Answer from the drawing. Dimensions are ordinates in mm from the lowest x, y and z of the part. A direction names the side the tool comes from. Coordinates: 2 decimals unless noted, no trailing zeros. Order: outer loops, then holes, each group sorted by start corner. A loop starts at its lowest first (then second) coordinate and runs counter-clockwise, first axis right, second up. Notation, with made-up numbers: (58.5, 7) - (73.5, 7) arc R26 cw to (73.5, 31) - close; hole circle Ø3 at (-13, -39.75). An arc over 180 degrees is marked (long way). Answer as a JSON object with one key per item and string values. Group by question number.
1) Find the intervals of material crossed by line 1 along X through (y, z) = (41, 22.5); line 2 along Y through (x, z) = (53.5, 13.75); line 3 along Y through (x, z) = (77, 10.5), in increasing order.
2) Section C-C (y = 30) is taken. Give the vertices of the cut face in (x, z), plus the area to 3 significant figures.
3) Section D-D (x = 12) is taken. Give the vertices of the cut face in (y, z), plus the area to 3 significant figures.
4) Each of these flat-tipped pins is pushed along its axis until it touches: P1, Ø6, axis at y = 51, z = 10.5, coming from the +X side; P2, Ø1.5, axis at x = 78, z = 7, coming from the +Y side; P3, Ø10, axis at x = 20.5, z = 18.5, coming from the +Y side. Where does it stop, or does it pass through?
5) A tool of negligible diameter and unlimited length cuts with its end or side. For the marked faces 1, 2 and 3, from which of +Z, -Z, +X, -X, +Y, -Y can it reach the whole face along a straight path? Write none if from no direction.
6) Section B-B (x = 44) is taken. Give the vertices of the cut face in (y, z).
7) Section A-A (z = 15) is taken. Give the vertices of the cut face in (x, y), plus the area to 3 significant figures.
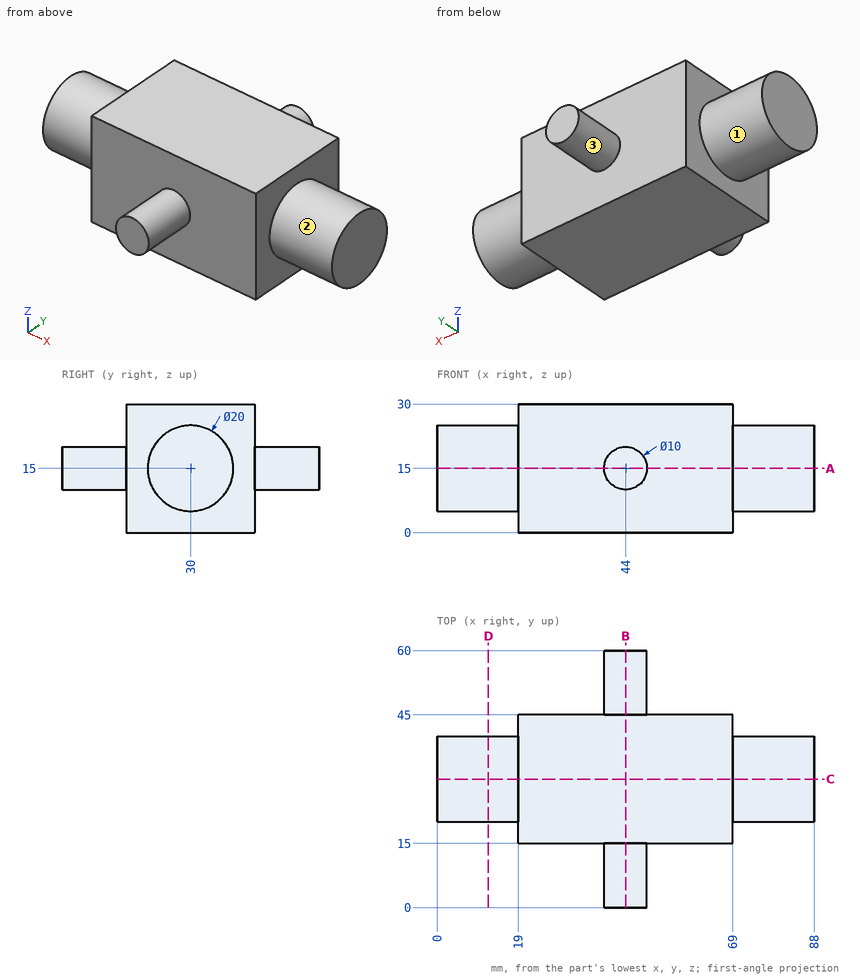
Report:
{
 "1": {"line 1": "x = 19 to 69", "line 2": "y = 15 to 45", "line 3": "y = 21.07 to 38.93"},
 "2": {"outline": "(0, 5) - (19, 5) - (19, 0) - (69, 0) - (69, 5) - (88, 5) - (88, 25) - (69, 25) - (69, 30) - (19, 30) - (19, 25) - (0, 25) - close", "area": "2,260 mm²"},
 "3": {"outline": "circle Ø20 at (30, 15)", "area": "314 mm²"},
 "4": {"P1": "stops at x = 48.77", "P2": "stops at y = 36.89", "P3": "stops at y = 45"},
 "5": {"face 1": "-X", "face 2": "+X", "face 3": "+Y"},
 "6": {"outline": "(0, 10) - (15, 10) - (15, 0) - (45, 0) - (45, 10) - (60, 10) - (60, 20) - (45, 20) - (45, 30) - (15, 30) - (15, 20) - (0, 20) - close"},
 "7": {"outline": "(0, 20) - (19, 20) - (19, 15) - (39, 15) - (39, 0) - (49, 0) - (49, 15) - (69, 15) - (69, 20) - (88, 20) - (88, 40) - (69, 40) - (69, 45) - (49, 45) - (49, 60) - (39, 60) - (39, 45) - (19, 45) - (19, 40) - (0, 40) - close", "area": "2,560 mm²"}
}
